The model under review builds one solid part; all positions refer to its coordinate system, in mm. A direction names the side the tool comes from. Coordinates: 2 decimals unless noted, no trailing zeros. Order: outer loops, then holes, each group sorted by start corner. A loop starts at its lowest first (then second) coordinate and runs counter-clockwise, first axis right, second up.
from build123d import *

# Parameters (mm, degrees)
SKETCH_W      = 800
SKETCH_H      = 500
PAD_DEPTH     = 850
SKETCH001_W   = 511.727677
SKETCH001_H   = 463.29253
PAD001_DEPTH  = 10
POCKET_DEPTH  = 220
SKETCH003_R   = 24.194915
PAD002_DEPTH  = 200
SKETCH004_W   = 56.527466
SKETCH004_H   = 197.218046
PAD003_DEPTH  = 20
SKETCH005_W   = 819.629583
SKETCH005_H   = 524.761626
SKETCH005_W_2 = 475.380982
SKETCH005_H_2 = 411.07835
PAD004_DEPTH  = 100
SKETCH006_W   = 769.3365
SKETCH006_H   = 11.482666
SKETCH006_W_2 = 764.743431
SKETCH006_H_2 = 9.186035
PAD005_DEPTH  = 10


with BuildPart() as part:
    # Sketch → Pad (new body)
    with BuildSketch(Plane.XZ):
        with Locations((400, 250)):
            Rectangle(SKETCH_W, SKETCH_H)
    extrude(amount=PAD_DEPTH)

    # Sketch001 (on Face5 of Pad) → Pad001 (join)
    with BuildSketch(Plane(origin=(0, 0, 0), x_dir=(1, 0, 0), z_dir=(0, 1, 0))):
        with Locations((400.552361, -244.345876)):
            Rectangle(SKETCH001_W, SKETCH001_H)
    extrude(amount=PAD001_DEPTH)

    # Sketch002 (on Face11 of Pad001) → Pocket (cut)
    with BuildSketch(Plane(origin=(0, 10, 0), x_dir=(1, 0, 0), z_dir=(0, 1, 0))):
        with BuildLine():
            Line((181.290512, -129.286423), (181.290512, -404.444153))
            ThreePointArc((181.290512, -404.444153), (195.935173, -439.799492), (231.290512, -454.444153))
            Line((231.290512, -454.444153), (577.500916, -454.444153))
            ThreePointArc((577.500916, -454.444153), (612.856255, -439.799492), (627.500916, -404.444153))
            Line((627.500916, -404.444153), (627.500916, -129.286423))
            ThreePointArc((627.500916, -129.286423), (612.856255, -93.931084), (577.500916, -79.286423))
            Line((577.500916, -79.286423), (231.290512, -79.286423))
            ThreePointArc((231.290512, -79.286423), (195.935173, -93.931084), (181.290512, -129.286423))
        make_face()
    extrude(amount=-POCKET_DEPTH, mode=Mode.SUBTRACT)

    # Sketch003 (on Face11 of Pocket) → Pad002 (join)
    with BuildSketch(Plane(origin=(0, 10, 0), x_dir=(1, 0, 0), z_dir=(0, 1, 0))):
        with Locations((399.065338, -48.817406)):
            Circle(SKETCH003_R)
    extrude(amount=PAD002_DEPTH)

    # Sketch004 (on Face21 of Pad002) → Pad003 (join)
    with BuildSketch(Plane(origin=(0, 210, 0), x_dir=(1, 0, 0), z_dir=(0, 1, 0))):
        with Locations((399.339508, -115.610719)):
            Rectangle(SKETCH004_W, SKETCH004_H)
    extrude(amount=PAD003_DEPTH)

    # Sketch005 (on Face4 of Pad003) → Pad004 (join)
    with BuildSketch(Plane(origin=(0, 0, 0), x_dir=(1, 0, 0), z_dir=(0, 1, 0))):
        with Locations((398.620938, -251.461533)):
            Rectangle(SKETCH005_W, SKETCH005_H)
        with Locations((403.098633, -266.965067)):
            Rectangle(SKETCH005_W_2, SKETCH005_H_2, mode=Mode.SUBTRACT)
    extrude(amount=-PAD004_DEPTH)

    # Sketch006 (on Face8 of Pad004) → Pad005 (join)
    with BuildSketch(Plane(origin=(0, 0, 500), x_dir=(-1, 0, 0), z_dir=(0, 0, 1))):
        with Locations((-400.80227, 350.871674)):
            Rectangle(SKETCH006_W, SKETCH006_H)
        with Locations((-400.802265, 627.603149)):
            Rectangle(SKETCH006_W_2, SKETCH006_H_2)
    extrude(amount=PAD005_DEPTH)


solid = part.part
(1) Consider section A-A (z = 158). Give the boundary of the cut face in (x, y).
(2) The part is to be moulded in two halves that separate along Y. For faces 5 (the face through (421.415, 108.6, 58.084)), 6 (the face through (394, -850, 254)), 7 (the face through (394, -470, 500)), 8 (the face through (-11.194, -49, 255)), say which applies: +Y half, -Y half, draft (parallel to the pull), parting line (faces both ways), or undercut.
(3) Consider section C-C (x = 555). Give the boundary of the cut face in (y, z), then the cut area to 3 significant figures.
(4) Tool access review of faces 1 (the face through (800, -470, 247)), 2 (the face through (394, -470, 0)), 3 (the face through (627.501, -98, 269)), 4 (the face through (393, -49, 513.842)): name each direction out of +Z, -Z, +X, -X, +Y, -Y from which nothing blocks a thin tool from reaching the whole face with its end or side.
(5) Insertion check: pin 1 Ø6 at (x, y) = (545.5, -393) entering from +Z; pin 2 Ø10 at (x, y) = (300.5, -226) entering from -Z; pin 3 Ø11 at (y, z) = (6, 156.5) entering from +X. Each pin has a flat end and moves straight along its axis. Give the tip position at first contact, or say it passes through.
(6) Consider section B-B (y = -38.5). Give the boundary of the cut face in (x, z).
(7) Consider section D-D (y = -399). Give the boundary of the cut face in (x, z).
(8) Wall thickness on line 1 (Z direction, x = 410.5, y = -58.5); line 2 (X direction, y = -320, z = 65); line 3 (Y direction, x = 431.5, z = 26): over which ranges is each line inside the solid? List them lowest first.
Findings:
1. outline: (-11.19, -100) - (0, -100) - (0, -850) - (800, -850) - (800, -100) - (808.44, -100) - (808.44, 0) - (656.42, 0) - (656.42, 10) - (627.5, 10) - (627.5, -210) - (181.29, -210) - (181.29, 10) - (144.69, 10) - (144.69, 0) - (-11.19, 0) - close; (371.08, 210) - (427.6, 210) - (427.6, 230) - (371.08, 230) - close
2. face 5: undercut
2. face 6: -Y half
2. face 7: undercut
2. face 8: draft
3. outline: (-850, 0) - (-100, 0) - (-100, -10.92) - (0, -10.92) - (0, 12.7) - (10, 12.7) - (10, 79.29) - (-210, 79.29) - (-210, 454.44) - (10, 454.44) - (10, 475.99) - (0, 475.99) - (0, 513.84) - (-100, 513.84) - (-100, 500) - (-345.13, 500) - (-345.13, 510) - (-356.61, 510) - (-356.61, 500) - (-623.01, 500) - (-623.01, 510) - (-632.2, 510) - (-632.2, 500) - (-850, 500) - close
3. area: 350,000 mm2
4. face 1: +Z, -Z, +X, -Y
4. face 2: -Z, +X, -X, -Y
4. face 3: +Y
4. face 4: +Z, +X, -X, +Y, -Y
5. pin 1: stops at z = 500
5. pin 2: stops at z = 0
5. pin 3: stops at x = 656.42
6. outline: (-11.19, -10.92) - (808.44, -10.92) - (808.44, 513.84) - (-11.19, 513.84) - close; hole (181.29, 129.29) arc R50 ccw to (231.29, 79.29) - (577.5, 79.29) arc R50 ccw to (627.5, 129.29) - (627.5, 404.44) arc R50 ccw to (577.5, 454.44) - (231.29, 454.44) arc R50 ccw to (181.29, 404.44) - close
7. outline: (0, 0) - (800, 0) - (800, 500) - (0, 500) - close
8. line 1: z = -10.92 to 79.29, 454.44 to 513.84
8. line 2: x = 0 to 800
8. line 3: y = -850 to 10
